from build123d import *

# Parameters (mm, degrees)
SKETCH1_W                       = 10.5664
SKETCH1_H                       = 7.5
BOSS_EXTRUDE1_DEPTH             = 20.5359
BOSS_EXTRUDE2_DEPTH             = 12.6492
SKETCH4_W                       = 7.9375
SKETCH4_H                       = 6.3373
F_21_0_159_DIAMETER_HOLE1_D     = 4.0386
F_21_0_159_DIAMETER_HOLE1_DEPTH = 15.875
F_21_0_159_DIAMETER_HOLE1_TIP   = 1.213317848
SKETCH7_R                       = 3.175
CUT_EXTRUDE1_DEPTH              = 12.7


with BuildPart() as part:
    # Sketch1 → Revolve1 (revolve)
    with BuildSketch(Plane.XY):
        with Locations((3.94335, 3.75)):
            Rectangle(SKETCH1_W, SKETCH1_H)
    revolve(axis=Axis((-1.33985, 0, 0), (1, 0, 0)))

    # Sketch2 → Boss-Extrude1 (add)
    with BuildSketch(Plane.ZY.offset(1.33985)):
        with BuildLine():
            Line((-2.590301913, 6.35), (2.590301913, 6.35))
            ThreePointArc((2.590301913, 6.35), (3.429, 5.939202219), (4.204110358, 5.41826726))
            Line((4.204110358, 5.41826726), (6.79441227, 0.93173274))
            ThreePointArc((6.79441227, 0.93173274), (6.858, 0), (6.79441227, -0.93173274))
            Line((6.79441227, -0.93173274), (4.204110358, -5.41826726))
            ThreePointArc((4.204110358, -5.41826726), (3.429, -5.939202219), (2.590301913, -6.35))
            Line((2.590301913, -6.35), (-2.590301913, -6.35))
            ThreePointArc((-2.590301913, -6.35), (-3.429, -5.939202219), (-4.204110358, -5.41826726))
            Line((-4.204110358, -5.41826726), (-6.79441227, -0.93173274))
            ThreePointArc((-6.79441227, -0.93173274), (-6.858, 0), (-6.79441227, 0.93173274))
            Line((-6.79441227, 0.93173274), (-4.204110358, 5.41826726))
            ThreePointArc((-4.204110358, 5.41826726), (-3.429, 5.939202219), (-2.590301913, 6.35))
        make_face()
    extrude(amount=BOSS_EXTRUDE1_DEPTH)

    # Sketch3 → Boss-Extrude2 (add)
    with BuildSketch(Plane(origin=(9.22655, 0, 0), x_dir=(0, 0, -1), z_dir=(1, 0, 0))):
        Polygon((3.666174209, -6.35), (-3.666174209, -6.35), (-7.332348419, 0), (-3.666174209, 6.35), (3.666174209, 6.35), (7.332348419, 0), align=None)
    extrude(amount=BOSS_EXTRUDE2_DEPTH)

    # Sketch4 → Revolve2 (revolve)
    with BuildSketch(Plane(origin=(0, 0, 0), x_dir=(-1, 0, 0), z_dir=(0, 0, -1))):
        with Locations((-25.8445, 3.16865)):
            Rectangle(SKETCH4_W, SKETCH4_H)
    revolve(axis=Axis((29.81325, 0, 0), (-1, 0, 0)))

    # #21 (0.159) Diameter Hole1
    with Locations(Plane.ZY.offset(21.87575)):
        with Locations((0, 0)):
            Hole(F_21_0_159_DIAMETER_HOLE1_D / 2, depth=F_21_0_159_DIAMETER_HOLE1_DEPTH)
            with Locations((0, 0, -(F_21_0_159_DIAMETER_HOLE1_DEPTH + F_21_0_159_DIAMETER_HOLE1_TIP / 2))):  # 118° drill point
                Cone(0, F_21_0_159_DIAMETER_HOLE1_D / 2, F_21_0_159_DIAMETER_HOLE1_TIP, mode=Mode.SUBTRACT)

    # Sketch7 → Cut-Extrude1 (cut)
    with BuildSketch(Plane.ZY.offset(21.87575)):
        Circle(SKETCH7_R)
    extrude(amount=-CUT_EXTRUDE1_DEPTH, mode=Mode.SUBTRACT)


solid = part.part
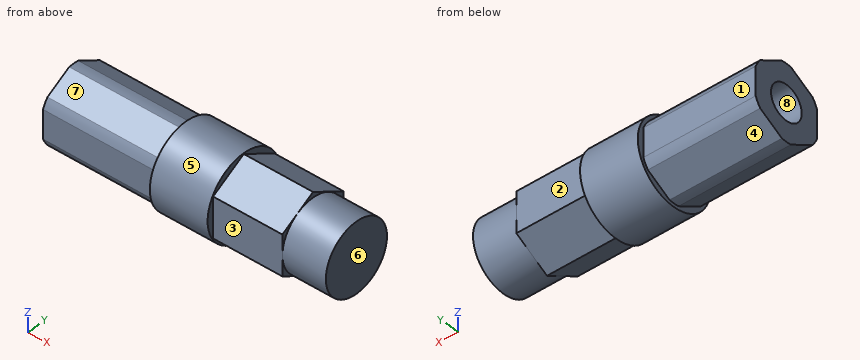
Can you work these out from the model? Positions are in its coordinate system, mm. Face numbers are marked on the shaded views. A direction names the side the tool comes from. Coordinates: 2 decimals unless noted, no trailing zeros. Write each loop counter-clockwise with the first axis right and the second up, starting at its lowest first coordinate (ties: lowest second). Pieces come first, ordered by that corner, then holes. Notation, with made-up numbers: (-5, 71) - (24, 71) arc R11 cw to (24, 90) - close; hole circle Ø5 at (-0.75, -16). An arc over 180 degrees is marked (long way). Return JSON: item names as keys, results as strings. Group by question number.
Item 1: Which directions (+Z, -Z, +X, -X, +Y, -Y) give clear straight access to the entire face, cutting with the end or side of a thin tool? Please do the marked faces 1, 2, 3 and 4.
Item 2: Please list where these lines run through material, in increasing order: probe 1 along Y at (x, z) = (-6.55, 0); probe 2 along Y at (x, z) = (-13.5, 0) (3 decimals); probe 3 along Z at (x, y) = (5.5, -4).
Item 3: We'd pull the mould along Z, two halves only. Please class the marked faces 5, 6, 7 and 8: pulls with the +Z half, pulls with the -Z half, needs draft (parallel to the pull), parting line crosses it, or undercut.
Item 4: If we section it at C-C (x = 3): Write out the boundary of the cut face in (y, z), then the cut area to 3 significant figures.
Item 5: If we section it at A-A (x = -14): Write out the boundary of the cut face in (y, z) (3 decimals).
Item 6: I'm going to push flat-ended pins straight in: pin 1 Ø2.5 at (x, z) = (-14, 1) entering from +Y; pin 2 Ø1.5 at (x, z) = (-15, 5.5) entering from +Y; pin 3 Ø4 at (x, z) = (-14.5, 0.5) entering from -Y. Where does each tip first touch, or does it pass through?
Item 7: If we section it at B-B (x = -6.5): Write out the boundary of the cut face in (y, z).
Return value:
{
 "1": {"face 1": "+Z, -Z, -X, +Y", "face 2": "+Z, -Z, +X, +Y", "face 3": "+Z, -Z, +X, -Y", "face 4": "-Z, -X, +Y"},
 "2": {"probe 1": "y = -6.35 to -2.02, 2.02 to 6.35", "probe 2": "y = -6.35 to -3.175, 3.175 to 6.35", "probe 3": "z = -6.34 to 6.34"},
 "3": {"face 5": "parting line crosses it", "face 6": "needs draft", "face 7": "pulls with the +Z half", "face 8": "undercut"},
 "4": {"outline": "circle Ø15 at (0, 0)", "area": "177 mm^2"},
 "5": {"outline": "(-6.35, -2.59) arc R6.858 ccw to (-5.418, -4.204) - (-0.932, -6.794) arc R6.858 ccw to (0.932, -6.794) - (5.418, -4.204) arc R6.858 ccw to (6.35, -2.59) - (6.35, 2.59) arc R6.858 ccw to (5.418, 4.204) - (0.932, 6.794) arc R6.858 ccw to (-0.932, 6.794) - (-5.418, 4.204) arc R6.858 ccw to (-6.35, 2.59) - close; hole circle Ø6.35 at (0, 0)"},
 "6": {"pin 1": "stops at y = 6.35", "pin 2": "stops at y = 4.47", "pin 3": "stops at y = -6.35"},
 "7": {"outline": "(-6.35, -2.59) arc R6.86 ccw to (-5.42, -4.2) - (-0.93, -6.79) arc R6.86 ccw to (0.93, -6.79) - (5.42, -4.2) arc R6.86 ccw to (6.35, -2.59) - (6.35, 2.59) arc R6.86 ccw to (5.42, 4.2) - (0.93, 6.79) arc R6.86 ccw to (-0.93, 6.79) - (-5.42, 4.2) arc R6.86 ccw to (-6.35, 2.59) - close; hole circle Ø4.04 at (0, 0)"}
}
